Input: dimensioned drawing with shaded views. Units: mm. Origin: part minimum x, y, z. Coordinates: 2 decimals unless noted, no trailing zeros. Loops run counter-clockwise (first coordinate to the right, second up) from the corner with the lowest first, then second, coordinate; pieces in that order, holes last. Notation, with made-up numbers: (-5.75, 11.25) - (15.25, 11.25) arc R17 cw to (15.25, 18.25) - close; hole circle Ø4 at (44.25, 68.25). An arc over 180 degrees is marked (long way). Put each result on its own line as item: value. Start each with the question number.
1) Section B-B on y = 221.5. Output: boundary loops of the cut face in (x, z).
2) Contact query for flat-ended pins moving along their axis: pin 1 Ø1.5 at (x, z) = (115, 8) entering from +Y; pin 2 Ø9 at (x, y) = (335, 159) entering from -Z; pin 3 Ø1.5 at (x, z) = (368, 2) entering from -Y. Output: stop coordinate, or through.
3) Material intervals for line 1 along Y through (x, z) = (461, 13.25); line 2 along X through (y, z) = (159, 4.5); line 3 along Y through (x, z) = (427, 6.5), sorted ascending. Write a range as from..to.
4) Section A-A on z = 5.5. Output: boundary loops of the cut face in (x, y), and give its area (3 significant figures).
5) Section C-C on x = 110. Output: boundary loops of the cut face in (y, z).
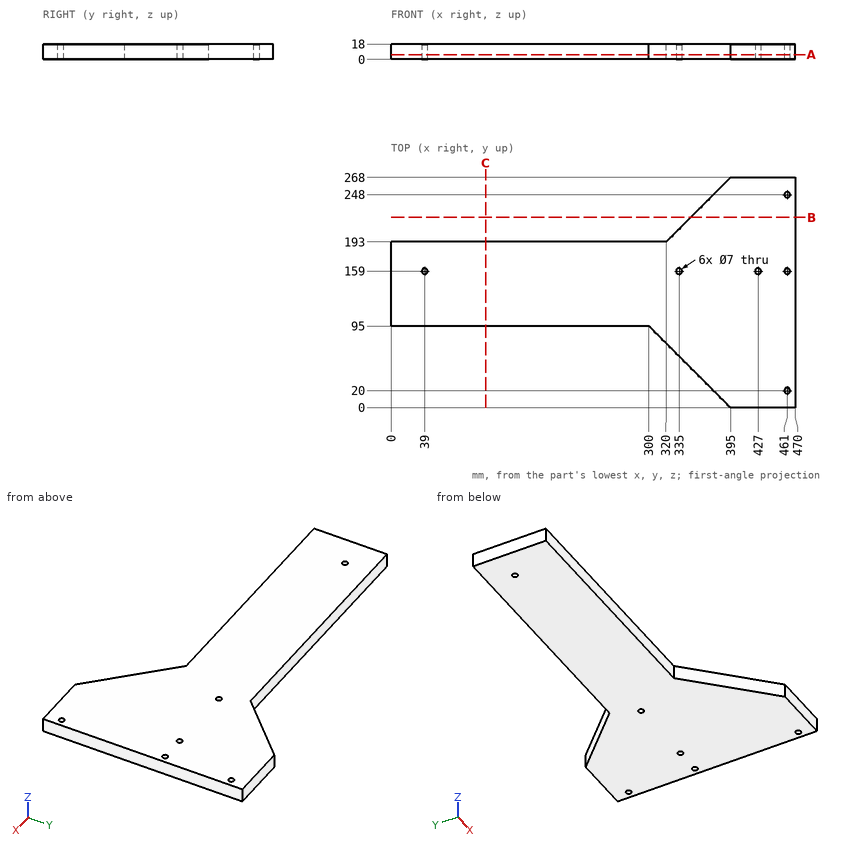
Answer block:
1. outline: (348.5, 0) - (470, 0) - (470, 18) - (348.5, 18) - close
2. pin 1: stops at y = 193
2. pin 2: stops at z = 0
2. pin 3: stops at y = 26.25
3. line 1: y = 0..16.5, 23.5..155.5, 162.5..244.5, 251.5..268
3. line 2: x = 0..35.5, 42.5..331.5, 338.5..423.5, 430.5..457.5, 464.5..470
3. line 3: y = 0..155.5, 162.5..268
4. outline: (0, 95) - (300, 95) - (395, 0) - (470, 0) - (470, 268) - (395, 268) - (320, 193) - (0, 193) - close; hole circle Ø7 at (39, 159); hole circle Ø7 at (335, 159); hole circle Ø7 at (427, 159); hole circle Ø7 at (461, 20); hole circle Ø7 at (461, 159); hole circle Ø7 at (461, 248)
4. area: 65,900 mm²
5. outline: (95, 0) - (193, 0) - (193, 18) - (95, 18) - close
